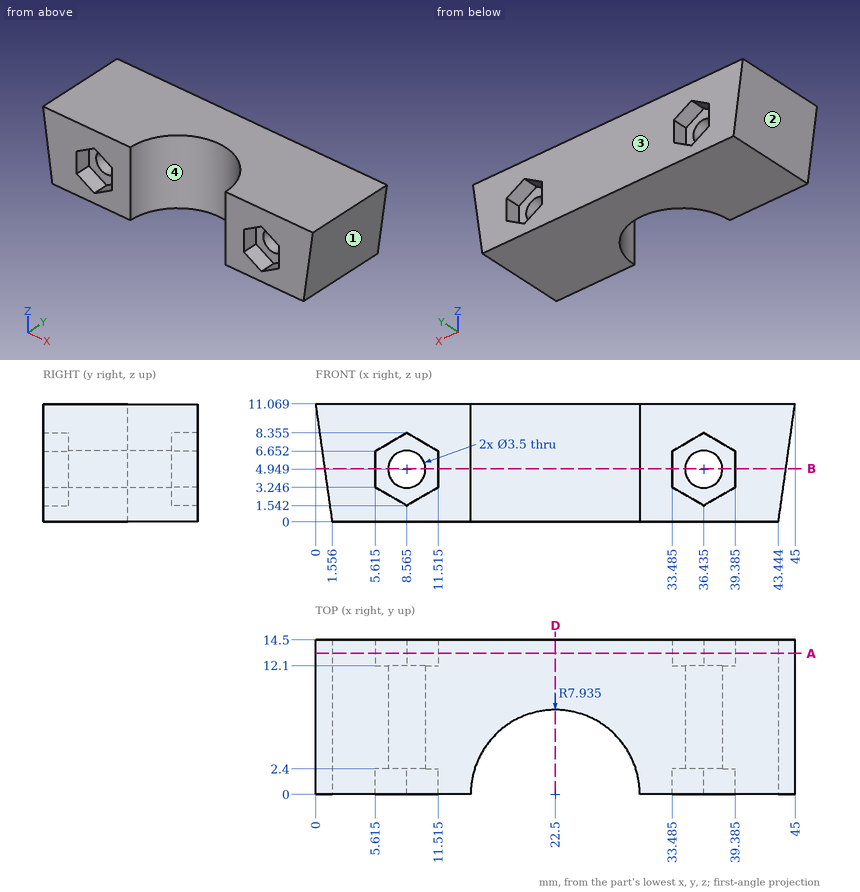
Geometry check sheet. Reference: drawing and pictorial views, mm from the part's lowest x, y, z. Round coordinates to 2 decimals unless told otherwise and drop trailing zeros. Order: outer loops, then holes, each group sorted by start corner. A loop starts at its lowest first (then second) coordinate and runs counter-clockwise, first axis right, second up. Notation, with made-up numbers: M 50,-11 L 58,-11 A21 cw 58,4 Z; hole C -28,6 d5. An arc over 180 degrees is marked long. Answer in a Markdown table with one row per item.
(1) Sectioned sample at B-B, the plane z = 5. State how many separate pieces and enclosed holes the cut face has, and give its area (3 significant figures).
Responses:
| item | result |
|---|---|
| separate pieces | 3 |
| enclosed holes | 0 |
| area | 404 mm² |
(2) Draft check along X on the marked faces 1, 2, 3 and 4. Enter one of: released by +X, released by -X, zero draft, split by the parting line, or undercut.
Responses:
| item | result |
|---|---|
| face 1 | released by +X |
| face 2 | released by -X |
| face 3 | zero draft |
| face 4 | undercut |
(3) Sectioned sample at A-A, the plane y = 13.25. Record the cut outline in (x, z) (1 decimal).
Responses:
| item | result |
|---|---|
| outline | M 0,11.1 L 1.6,0 L 43.4,0 L 45,11.1 Z; hole M 5.6,3.2 L 8.6,1.5 L 11.5,3.2 L 11.5,6.7 L 8.6,8.4 L 5.6,6.7 Z; hole M 33.5,3.2 L 36.4,1.5 L 39.4,3.2 L 39.4,6.7 L 36.4,8.4 L 33.5,6.7 Z |
(4) Go/stop test with flat-tipped pins: P1, Ø1.2, axis at y = 1, z = 4, coming from the +X side; P2, Ø5, axis at y = 4.5, z = 6, coming from the -X side; P3, Ø6.5, axis at x = 9, z = 6, coming from the -Y side; P4, Ø2, axis at x = 20, z = 6, coming from the -Y side. Record where each tip stops, or that it passes through.
Responses:
| item | result |
|---|---|
| P1 | stops at x = 44.09 |
| P2 | stops at x = 0.36 |
| P3 | stops at y = 0 |
| P4 | stops at y = 7.12 |
(5) Sectioned sample at D-D, the plane x = 22.5. Record the cut outline in (y, z) (1 decimal).
Responses:
| item | result |
|---|---|
| outline | M 7.9,0 L 14.5,0 L 14.5,11.1 L 7.9,11.1 Z |
(6) Scan lines: probe 1 along X at (y, z) = (2.5, 5.25); probe 2 along X at (y, z) = (5.5, 5.25); probe 3 along X at (y, z) = (4.5, 10.75) (1 decimal). Record each from-to range of solid material in increasing order. Write a range as from..to.
Responses:
| item | result |
|---|---|
| probe 1 | x = 0.82..6.84, 10.29..14.97, 30.03..34.71, 38.16..44.18 |
| probe 2 | x = 0.82..6.84, 10.29..16.78, 28.22..34.71, 38.16..44.18 |
| probe 3 | x = 0..16, 29..45 |
